Verification items for the finished model (mm, model axes). A direction names the side the tool comes from. Give positions to 0.01 mm unless a question says otherwise; leave off trailing zeros. Order: outer loops, then holes, each group sorted by start corner. A loop starts at its lowest first (then second) coordinate and runs counter-clockwise, first axis right, second up.
from build123d import *

# Parameters (mm, degrees)
SKETCH_W      = 17.25
SKETCH_H      = 10
PAD_DEPTH     = 1.5
SKETCH001_W   = 17.25
SKETCH001_H   = 10
SKETCH001_W_2 = 14.25
SKETCH001_H_2 = 7
PAD001_DEPTH  = 50
SKETCH002_R   = 6.1
POCKET_DEPTH  = 1.5
SKETCH003_W   = 17.25
SKETCH003_H   = 10
SKETCH003_W_2 = 12.05
SKETCH003_H_2 = 4.55
PAD002_DEPTH  = 1.5


with BuildPart() as part:
    # Sketch → Pad (new body)
    with BuildSketch(Plane.XY):
        Rectangle(SKETCH_W, SKETCH_H)
    extrude(amount=PAD_DEPTH)

    # Sketch001 (on Face6 of Pad) → Pad001 (join)
    with BuildSketch(Plane.XY.offset(1.5)):
        Rectangle(SKETCH001_W, SKETCH001_H)
        Rectangle(SKETCH001_W_2, SKETCH001_H_2, mode=Mode.SUBTRACT)
    extrude(amount=PAD001_DEPTH)

    # Sketch002 (on Face6 of Pad001) → Pocket (cut)
    with BuildSketch(Plane(origin=(0, 5, 0), x_dir=(-1, 0, 0), z_dir=(0, 1, 0))):
        with Locations((0, 7.5)):
            Circle(SKETCH002_R)
    extrude(amount=-POCKET_DEPTH, mode=Mode.SUBTRACT)

    # Sketch003 (on Face11 of Pocket) → Pad002 (join)
    with BuildSketch(Plane.XY.offset(51.5)):
        Rectangle(SKETCH003_W, SKETCH003_H)
        with Locations((0, 0.375)):
            Rectangle(SKETCH003_W_2, SKETCH003_H_2, mode=Mode.SUBTRACT)
    extrude(amount=PAD002_DEPTH)


solid = part.part
(1) Section check C-C, the plane z = 37.5. Enter the section's corners in (x, y) (3 decimals), then the cut area to 4 significant figures.
Solved:
outline: (-8.625, -5) - (8.625, -5) - (8.625, 5) - (-8.625, 5) - close; hole (-7.125, -3.5) - (7.125, -3.5) - (7.125, 3.5) - (-7.125, 3.5) - close
area: 72.75 mm2
(2) Set-up check for faces 4 (the cylindrical face through (1.322, 4.26, 1.545)), 5 (the flat face through (-0.1, -2.3, 51.5)), 6 (the flat face through (0, -5, 26)), 7 (the flat face through (6.025, 0, 52)), 8 (the flat face through (0, 0, 0)): record each of +Z, -Z, +X, -X, +Y, -Y from which the full face is reachable in a straight line by a thin tool's end or side.
Solved:
face 4: +Y
face 5: none
face 6: +Z, -Z, +X, -X, -Y
face 7: +Z
face 8: -Z, +X, -X, +Y, -Y
(3) Section check B-B, the plane x = 0. Enter the section's corners in (y, z), then the cut area to 3 significant figures.
Solved:
outline: (-5, 0) - (5, 0) - (5, 1.4) - (3.5, 1.4) - (3.5, 1.5) - (-3.5, 1.5) - (-3.5, 51.5) - (-1.9, 51.5) - (-1.9, 53) - (-5, 53) - close; (2.65, 51.5) - (3.5, 51.5) - (3.5, 13.6) - (5, 13.6) - (5, 53) - (2.65, 53) - close
area: 155 mm2
(4) Section check A-A, the plane y = -2.5. Enter the section's corners in (x, z) (3 decimals), then the cut area to 3 significant figures.
Solved:
outline: (-8.625, 0) - (8.625, 0) - (8.625, 53) - (-8.625, 53) - close; hole (-7.125, 1.5) - (7.125, 1.5) - (7.125, 51.5) - (-7.125, 51.5) - close
area: 202 mm2
(5) Scan lines: line 1 (Z direction, x = 0, y = 4.2); line 2 (Z direction, x = 5.5, y = 3); line 3 (Y direction, x = -1.5, z = 19). Record each from-to range of solid material in increasing order.
Solved:
line 1: z = 0 to 1.4, 13.6 to 53
line 2: z = 0 to 1.5, 51.5 to 53
line 3: y = -5 to -3.5, 3.5 to 5
(6) Go/stop test with a flat-tipped pin: pin 1 (1 mm diameter, centred on x = -0.5, z = 7, fed in from +Y). Record where the tip stops, or that it passes through.
Solved:
pin 1: stops at y = -3.5
(7) Section check D-D, the plane z = 7.5. Enter the section's corners in (x, y) (3 decimals).
Solved:
outline: (-8.625, -5) - (8.625, -5) - (8.625, 5) - (6.1, 5) - (6.1, 3.5) - (7.125, 3.5) - (7.125, -3.5) - (-7.125, -3.5) - (-7.125, 3.5) - (-6.1, 3.5) - (-6.1, 5) - (-8.625, 5) - close
(8) Release check for a two-part mould opening along Z. For faces 1 (the flat face through (0, -1.9, 52)), 2 (the flat face through (-0.1, -2.2, 53)), 3 (the flat face through (7.125, 0, 26)) record: pulls with the +Z half, pulls with the -Z half, needs draft (parallel to the pull), parting line crosses it, or undercut.
Solved:
face 1: needs draft
face 2: pulls with the +Z half
face 3: undercut
